Part model, mm, in its own coordinate system. Round coordinates to 2 decimals unless told otherwise and drop trailing zeros. Loops run counter-clockwise (first coordinate to the right, second up) from the corner with the lowest first, then second, coordinate; pieces in that order, holes last. Notation, with made-up numbers: M -19,56.5 L 8,56.5 A30 cw 8,78.5 Z; hole C 60.5,3.25 d8. An arc over 180 degrees is marked long. Answer as CSV lines item,"result". Start each with the question number.
Item 1: Wall check: line 1 (Z direction, x = 33.5, y = -1521); line 2 (Y direction, x = 32.5, z = 120); line 3 (Y direction, x = 32, z = 123). Give the ranges that are in metal, low to high.
Item 2: Drop flat-ended pins along their axis: pin 1 Ø16 at (x, y) = (32.5, -350) entering from +Z; pin 2 Ø1 at (y, z) = (-1195.5, 37) entering from +X. Give the stop position or say it passes through.
Item 3: Band-saw the part on A-A (y = -1272). Give the cut face in (x, z).
Item 4: Band-saw the part on B-B (z = 64). Give the cut face in (x, y), and give its area (3 significant figures).
```python
from build123d import *

# Parameters (mm, degrees)
F1_DEPTH = 1780
F3_DEPTH = 125.001
F5_DEPTH = 65.001
F6_R     = 9
F7_DEPTH = 7.5
F8_R     = 9
F9_DEPTH = 7.5


with BuildPart() as f1:
    # F0 (on Front) → F1 (new body)
    with BuildSketch(Plane.XZ):
        with BuildLine():
            Line((0, 125), (0, 0))
            Line((0, 0), (65, 0))
            Line((65, 0), (65, 7.5))
            Line((65, 7.5), (12.7, 7.5))
            ThreePointArc((12.7, 7.5), (7.043146, 9.843146), (4.7, 15.5))
            Line((4.7, 15.5), (4.7, 109.5))
            ThreePointArc((4.7, 109.5), (7.043146, 115.156854), (12.7, 117.5))
            Line((12.7, 117.5), (65, 117.5))
            Line((65, 117.5), (65, 125))
            Line((65, 125), (0, 125))
        make_face()
    extrude(amount=F1_DEPTH)

    # F2 (on face) → F3 (cut, through all)
    with BuildSketch(Plane.XY.offset(125)):
        Polygon((65, -65), (65, 0), (0, 0), align=None)
    extrude(amount=-F3_DEPTH, mode=Mode.SUBTRACT)

    # F4 (on face) → F5 (cut, through all)
    with BuildSketch(Plane(origin=(0, 0, 0), x_dir=(0, -1, 0), z_dir=(-1, 0, 0))):
        Polygon((1780, 0), (1780, 125), (1655, 125), align=None)
    extrude(amount=-F5_DEPTH, mode=Mode.SUBTRACT)

    # F6 (on face) → F7 (cut, through all)
    with BuildSketch(Plane.XY.offset(125)):
        with Locations((32.5, -350)):
            Circle(F6_R)
        with Locations((32.5, -452)):
            Circle(F6_R)
    extrude(amount=-F7_DEPTH, mode=Mode.SUBTRACT)

    # F8 (on face) → F9 (cut, through all)
    with BuildSketch(Plane.XY.offset(125)):
        with Locations((32.5, -1378)):
            Circle(F8_R)
        with Locations((32.5, -1480)):
            Circle(F8_R)
    extrude(amount=-F9_DEPTH, mode=Mode.SUBTRACT)


solid = f1.part
```
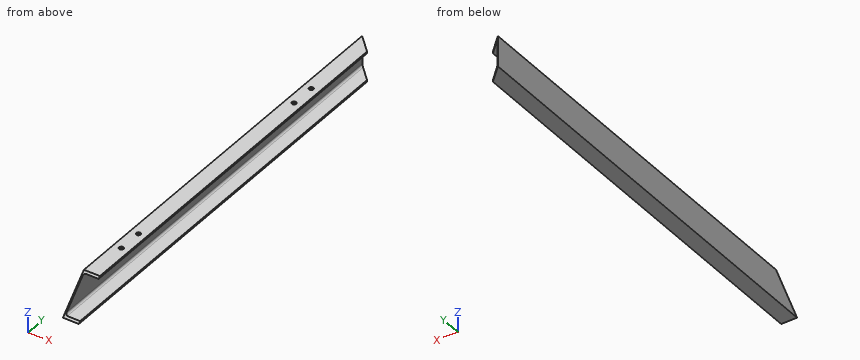
Answer block:
1,line 1,"z = 0 to 7.5, 117.5 to 125"
1,line 2,"y = -1660 to -1489, -1471 to -1387, -1369 to -461, -443 to -359, -341 to -32.5"
1,line 3,"y = -1657 to -1488.99, -1471.01 to -1386.99, -1369.01 to -460.99, -443.01 to -358.99, -341.01 to -32"
2,pin 1,"stops at z = 7.5"
2,pin 2,"stops at x = 4.7"
3,outline,"M 0,0 L 65,0 L 65,7.5 L 12.7,7.5 A8 cw 4.7,15.5 L 4.7,109.5 A8 cw 12.7,117.5 L 65,117.5 L 65,125 L 0,125 Z"
4,outline,"M 0,-1716 L 4.7,-1716 L 4.7,-4.7 L 0,0 Z"
4,area,"8,050 mm^2"
